Print and shaded views of the part. All mm, measured from the part's lowest x, y and z. Coordinates: 2 decimals unless noted, no trailing zeros. Order: outer loops, then holes, each group sorted by start corner. A loop starts at its lowest first (then second) coordinate and runs counter-clockwise, first axis right, second up.
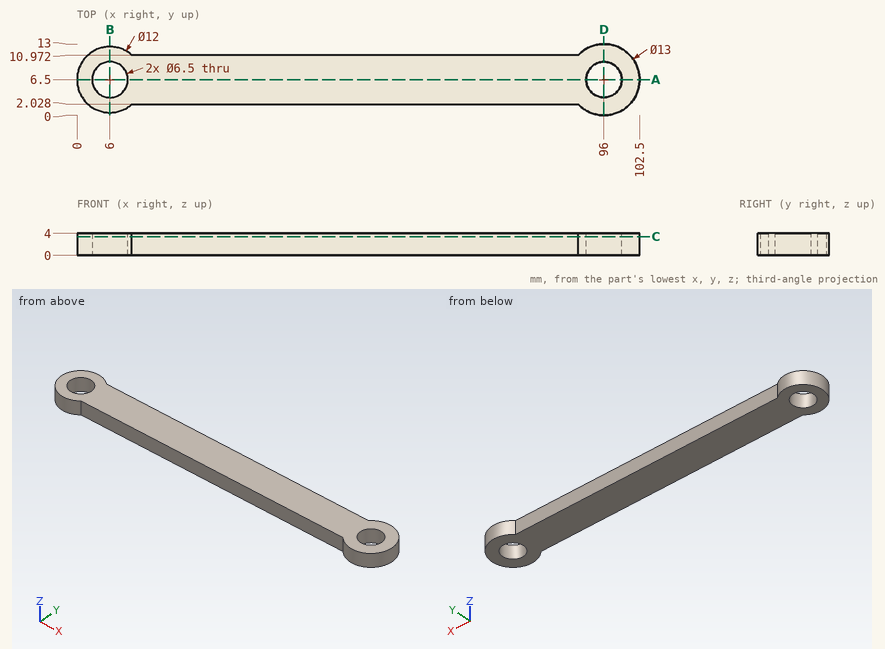
Q1. Cut at C-C, the plane z = 3.4. List the corners of the cut face in (x, y).
Established:
outline: (10, 2.03) - (91.28, 2.03) arc R6.5 ccw (long way) to (91.28, 10.97) - (10, 10.97) arc R6 ccw (long way) to start; hole circle Ø6.5 at (6, 6.5); hole circle Ø6.5 at (96, 6.5)
Q2. Probe line 1 (X direction, y = 5.25, z = 2.45); line 2 (X direction, y = 5.75, z = 3.05); line 3 (Y direction, x = 86, z = 1.1). List the from-to ranges inside material, lowest first.
Established:
line 1: x = 0.13 to 3, 9 to 93, 99 to 102.38
line 2: x = 0.05 to 2.84, 9.16 to 92.84, 99.16 to 102.46
line 3: y = 2.03 to 10.97
Q3. Drop flat-ended pins along their axis: P1, Ø1, axis at y = 10, z = 1.5, coming from the -X side; P2, Ø1, axis at y = 5, z = 2, coming from the +X side; P3, Ø1, axis at y = 4.5, z = 3, coming from the -X side. Give the stop position or say it passes through.
Established:
P1: stops at x = 0.8
P2: stops at x = 102.42
P3: stops at x = 0.19
Q4. Cut at B-B, the plane x = 6. List the corners of the cut face in (y, z), plus the area to 3 significant figures.
Established:
outline: (0.5, 0) - (3.25, 0) - (3.25, 4) - (0.5, 4) - close; (9.75, 0) - (12.5, 0) - (12.5, 4) - (9.75, 4) - close
area: 22.0 mm2
Q5. Cut at A-A, the plane y = 6.5. List the corners of the cut face in (x, z).
Established:
outline: (0, 0) - (2.75, 0) - (2.75, 4) - (0, 4) - close; (9.25, 0) - (92.75, 0) - (92.75, 4) - (9.25, 4) - close; (99.25, 0) - (102.5, 0) - (102.5, 4) - (99.25, 4) - close
Q6. Cut at D-D, the plane x = 96. List the corners of the cut face in (y, z), plus the area to 3 significant figures.
Established:
outline: (0, 0) - (3.25, 0) - (3.25, 4) - (0, 4) - close; (9.75, 0) - (13, 0) - (13, 4) - (9.75, 4) - close
area: 26.0 mm2
